Check sheet for the modelled part. Datum: model origin and axes. Units: mm. Face numbers are marked on the shaded views. A direction names the side the tool comes from. Round coordinates to 2 decimals unless told otherwise and drop trailing zeros. Loops run counter-clockwise (first coordinate to the right, second up) from the corner with the lowest first, then second, coordinate; pieces in that order, holes last. Notation, with made-up numbers: (55, -19) - (104, -19) arc R7 ccw to (104, -6) - close; hole circle Ø11 at (89.5, 71.5). An arc over 180 degrees is marked (long way). Put each result on its own line as item: value.
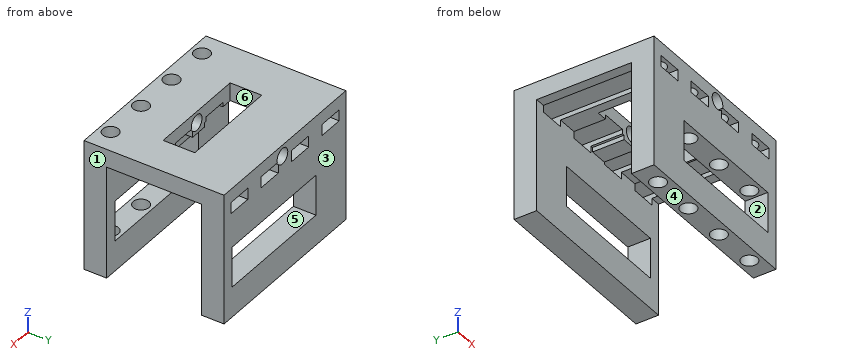
```python
from build123d import *

# Parameters (mm, degrees)
F0_W      = 48.3402396964
F0_H      = 20
F0_W_2    = 22
F0_H_2    = 7
F1_DEPTH  = 4
F3_DEPTH  = 1
F4_R      = 1.75
F5_DEPTH  = 20.001
F6_DEPTH  = 5.5
F7_DEPTH  = 5.5
F8_W      = 21.6701198482
F8_H      = 5
F9_DEPTH  = 25
F10_W     = 21.6701198482
F10_H     = 5
F11_DEPTH = 25
F12_W     = 5
F12_H     = 5
F13_DEPTH = 24
F14_W     = 5
F14_H     = 5
F15_DEPTH = 24
F16_W     = 11
F16_H     = 4.5
F17_DEPTH = 31.001
F19_DEPTH = 29.001
F18_R     = 1.75
F20_DEPTH = 10
F21_W     = 5.6
F21_H     = 2.5
F22_DEPTH = 31.001
F23_DEPTH = 29.001


# Not quite as in the source:
# - a feature names something its author has since deleted; it is built from what else it names


with BuildPart() as f1:
    # F0 (on Top) → F1 (new body)
    with BuildSketch(Plane.XY):
        with Locations((3.7882691845, -5.1383437738)):
            Rectangle(F0_W, F0_H)
        with Locations((3.7882691845, -5.1383437738)):
            Rectangle(F0_W_2, F0_H_2, mode=Mode.SUBTRACT)
    extrude(amount=F1_DEPTH)

    # F2 (on face) → F3 (join)
    with BuildSketch(Plane(origin=(0, 0, 0), x_dir=(1, 0, 0), z_dir=(0, 0, -1))):
        Polygon((6.2882691845, 1.6383437738), (3.7882691845, 1.6383437738), (1.2882691845, 1.6383437738), (1.2882691845, -4.8616562262), (6.2882691845, -4.8616562262), align=None)
        Polygon((1.2882691845, 8.6383437738), (3.7882691845, 8.6383437738), (6.2882691845, 8.6383437738), (6.2882691845, 15.1383437738), (1.2882691845, 15.1383437738), align=None)
    extrude(amount=F3_DEPTH)

    # F4 (on face) → F5 (cut, through all)
    with BuildSketch(Plane.XZ.offset(15.1383437738)):
        with Locations((3.7882691845, 1.5)):
            Circle(F4_R)
    extrude(amount=-F5_DEPTH, mode=Mode.SUBTRACT)

    # F6 (add): a face of the model
    f6_faces = [f1.faces().sort_by_distance(p)[0] for p in [
        (-19.8958693087, -15.1383437738, 2),
    ]]
    extrude(f6_faces, amount=F6_DEPTH)

    # F7 (add): a face of the model
    f7_faces = [f1.faces().sort_by_distance(p)[0] for p in [
        (27.4724076777, 4.8616562262, 2),
    ]]
    extrude(f7_faces, amount=F7_DEPTH)

    # F8 (on face) → F9 (join)
    with BuildSketch(Plane(origin=(0, 0, 0), x_dir=(1, 0, 0), z_dir=(0, 0, -1))):
        with Locations((17.1233291086, -7.8616562262)):
            Rectangle(F8_W, F8_H)
        with Locations((17.1233291086, 18.1383437738)):
            Rectangle(F8_W, F8_H)
    extrude(amount=F9_DEPTH)

    # F10 (on face) → F11 (join)
    with BuildSketch(Plane(origin=(0, 0, 0), x_dir=(1, 0, 0), z_dir=(0, 0, -1))):
        with Locations((-9.5467907396, 18.1383437738)):
            Rectangle(F10_W, F10_H)
        with Locations((-9.5467907396, -7.8616562262)):
            Rectangle(F10_W, F10_H)
    extrude(amount=F11_DEPTH)

    # F12 (on face) → F13 (join)
    with BuildSketch(Plane(origin=(0, 0, -1), x_dir=(1, 0, 0), z_dir=(0, 0, -1))):
        with Locations((3.7882691845, 18.1383437738)):
            Rectangle(F12_W, F12_H)
    extrude(amount=F13_DEPTH)

    # F14 (on face) → F15 (join)
    with BuildSketch(Plane(origin=(0, 0, -1), x_dir=(1, 0, 0), z_dir=(0, 0, -1))):
        with Locations((3.7882691845, -7.8616562262)):
            Rectangle(F14_W, F14_H)
    extrude(amount=F15_DEPTH)

    # F16 (on face) → F17 (cut, through all)
    with BuildSketch(Plane.XZ.offset(20.6383437738)):
        with Locations((9.2882691845, -16)):
            Rectangle(F16_W, F16_H)
        Polygon((3.7882691845, -18.25), (3.7882691845, -13.75), (14.7882691845, -13.75), (14.7882691845, -9.25), (-7.2117308155, -9.25), (-7.2117308155, -18.25), align=None)
        Polygon((14.7882691845, -9.25), (14.7882691845, -13.75), (14.7882691845, -18.25), (20.2882691845, -18.25), (20.2882691845, -9.25), align=None)
    extrude(amount=-F17_DEPTH, mode=Mode.SUBTRACT)

    # F18 (on face) → F19 (cut, through all)
    with BuildSketch(Plane.XY.offset(4)):
        Polygon((-20.3818506637, -20.6383437738), (-17.0416109673, -20.6383437738), (-17.0416109673, -5.1383437738), (-17.0416109673, 10.3616562262), (-20.3818506637, 10.3616562262), align=None)
    extrude(amount=-F19_DEPTH, mode=Mode.SUBTRACT)

    # F18 (on face) → F20 (cut)
    with BuildSketch(Plane.XY.offset(4)):
        with Locations((-12.0416109673, -18.1383437738)):
            Circle(F18_R)
    extrude(amount=-F20_DEPTH, mode=Mode.SUBTRACT)

    # F21 (on face) → F22 (cut, through all)
    with BuildSketch(Plane.XZ.offset(20.6383437738)):
        Polygon((-12.0416109673, 1), (-14.8416109673, 1), (-14.8416109673, -1.5), (-9.2416109673, -1.5), (-9.2416109673, 1), align=None)
        Polygon((27.9583890327, 4), (22.9583890327, 4), (22.9583890327, 1), (22.9583890327, -25), (27.9583890327, -25), align=None)
        with Locations((-2.0416109673, -0.25)):
            Rectangle(F21_W, F21_H)
        with BuildLine():
            Line((5.1583890327, 0.4112982035), (5.1583890327, -1.5))
            Line((5.1583890327, -1.5), (10.7583890327, -1.5))
            Line((10.7583890327, -1.5), (10.7583890327, 1))
            Line((10.7583890327, 1), (5.4653201677, 1))
            ThreePointArc((5.4653201677, 1), (5.3400278546, 0.6909604275), (5.1583890327, 0.4112982035))
        make_face()
        Polygon((20.7583890327, -1.5), (20.7583890327, 1), (17.9583890327, 1), (15.1583890327, 1), (15.1583890327, -1.5), align=None)
    extrude(amount=-F22_DEPTH, mode=Mode.SUBTRACT)

    # F18 (on face) → F23 (cut, through all)
    with BuildSketch(Plane.XY.offset(4)):
        Polygon((-17.0416109673, -20.6383437738), (-17.0416109673, -5.1383437738), (-17.0416109673, 10.3616562262), (-20.3818506637, 10.3616562262), (-20.3818506637, -20.6383437738), align=None)
        with Locations((-12.0416109673, -18.1383437738)):
            Circle(F18_R)
        with BuildLine():
            ThreePointArc((19.7083890327, -18.1383437738), (17.9583890327, -16.3883437738), (16.2083890327, -18.1383437738))
            ThreePointArc((16.2083890327, -18.1383437738), (17.9583890327, -19.8883437738), (19.7083890327, -18.1383437738))
        make_face()
        with BuildLine():
            ThreePointArc((9.7083890327, -18.1383437738), (7.9583890327, -16.3883437738), (6.2083890327, -18.1383437738))
            Line((6.2083890327, -18.1383437738), (7.9583890327, -18.1383437738))
            Line((7.9583890327, -18.1383437738), (9.7083890327, -18.1383437738))
        make_face()
        with BuildLine():
            Line((7.9583890327, -18.1383437738), (6.2083890327, -18.1383437738))
            ThreePointArc((6.2083890327, -18.1383437738), (7.9583890327, -19.8883437738), (9.7083890327, -18.1383437738))
            Line((9.7083890327, -18.1383437738), (7.9583890327, -18.1383437738))
        make_face()
        with BuildLine():
            ThreePointArc((-0.2916109673, -18.1383437738), (-2.0416109673, -16.3883437738), (-3.7916109673, -18.1383437738))
            Line((-3.7916109673, -18.1383437738), (-2.0416109673, -18.1383437738))
            Line((-2.0416109673, -18.1383437738), (-0.2916109673, -18.1383437738))
        make_face()
        with BuildLine():
            Line((-2.0416109673, -18.1383437738), (-3.7916109673, -18.1383437738))
            ThreePointArc((-3.7916109673, -18.1383437738), (-2.0416109673, -19.8883437738), (-0.2916109673, -18.1383437738))
            Line((-0.2916109673, -18.1383437738), (-2.0416109673, -18.1383437738))
        make_face()
    extrude(amount=-F23_DEPTH, mode=Mode.SUBTRACT)


solid = f1.part
```
Item 1: Thickness scan on line 1 (Z direction, x = -2, y = 5.5); line 2 (Y direction, x = 13, z = -22.75); line 3 (Z direction, x = -14.5, y = -16.5). Record the ranges inside material, lowest first. Write a range as from..to.
Filled sheet:
line 1: -25..-18.25, -9.25..-1.5, 1..4
line 2: -20.64..-15.64, 5.36..10.36
line 3: -25..-1.5, 1..4
Item 2: Tool access check on the marked faces 4, 5 and 6. Record the directions out of +Z, -Z, +X, -X, +Y, -Y that give a thin tool (end or side, any length) a straight path to the whole face; none if there is none.
Filled sheet:
face 4: -Z, +X, -X, +Y, -Y
face 5: +Y, -Y
face 6: +Z, -Z
Item 3: Section check D-D on z = -19. Enter the section's corners in (x, y).
Filled sheet:
outline: (-17.04, -20.64) - (22.96, -20.64) - (22.96, -15.64) - (-17.04, -15.64) - close; (-17.04, 5.36) - (22.96, 5.36) - (22.96, 10.36) - (-17.04, 10.36) - close; hole circle Ø3.5 at (-12.04, -18.14); hole circle Ø3.5 at (-2.04, -18.14); hole circle Ø3.5 at (7.96, -18.14); hole circle Ø3.5 at (17.96, -18.14)
Item 4: Section check C-C on y = -11. Enter the section's corners in (x, z).
Filled sheet:
outline: (-17.04, 0) - (-14.84, 0) - (-14.84, 1) - (-9.24, 1) - (-9.24, 0) - (-4.84, 0) - (-4.84, 1) - (0.76, 1) - (0.76, 0) - (1.29, 0) - (1.29, -1) - (5.16, -1) - (5.16, 0.41) arc R1.75 cw (long way) to (5.47, 1) - (10.76, 1) - (10.76, 0) - (15.16, 0) - (15.16, 1) - (20.76, 1) - (20.76, 0) - (22.96, 0) - (22.96, 4) - (-17.04, 4) - close
Item 5: Section check A-A on z = 1.5. Enter the section's corners in (x, y), then the cut area to 3 significant figures.
Filled sheet:
outline: (-17.04, -20.64) - (2.04, -20.64) - (2.04, -8.64) - (-7.21, -8.64) - (-7.21, -1.64) - (2.04, -1.64) - (2.04, 10.36) - (-17.04, 10.36) - close; (5.54, -20.64) - (22.96, -20.64) - (22.96, 10.36) - (5.54, 10.36) - (5.54, -1.64) - (14.79, -1.64) - (14.79, -8.64) - (5.54, -8.64) - close; hole circle Ø3.5 at (-12.04, -18.14); hole circle Ø3.5 at (-2.04, -18.14); hole circle Ø3.5 at (7.96, -18.14); hole circle Ø3.5 at (17.96, -18.14)
area: 964 mm²
Item 6: Section check B-B on x = 11.5. Enter the section's corners in (y, z), then the cut area to 3 significant figures.
Filled sheet:
outline: (-20.64, -25) - (-15.64, -25) - (-15.64, -18.25) - (-20.64, -18.25) - close; (-20.64, -9.25) - (-15.64, -9.25) - (-15.64, 0) - (-8.64, 0) - (-8.64, 4) - (-20.64, 4) - close; (-1.64, 0) - (5.36, 0) - (5.36, -9.25) - (10.36, -9.25) - (10.36, 4) - (-1.64, 4) - close; (5.36, -25) - (10.36, -25) - (10.36, -18.25) - (5.36, -18.25) - close
area: 256 mm²
Item 7: Go/stop test with flat-tipped pins: pin 1 (12.5 mm diameter, centred on x = 0.5, z = -12.5, fed in from +Y); pin 2 (1.5 mm diameter, centred on x = -4.5, y = -3, fed in from +Z); pin 3 (3 mm diameter, centred on x = -11, y = -7.5, fed in from -Z); pin 4 (3.5 mm diameter, centred on x = 12, y = -9, fed in from -Z). Record where each tip stops, or that it passes through.
Filled sheet:
pin 1: y = 10.36
pin 2: through
pin 3: z = 1
pin 4: z = 0
Item 8: Release check for a two-part mould opening along X. For the marked faces 1, 2 and 3 record: +X half, -X half, draft (parallel to the pull), parting line (faces both ways), or undercut.
Filled sheet:
face 1: +X half
face 2: undercut
face 3: draft
